Model file for the job. Use its own axes, mm. A direction names the side the tool comes from. Coordinates: 2 decimals unless noted, no trailing zeros. Order: outer loops, then holes, each group sorted by start corner. A loop starts at its lowest first (then second) coordinate and runs counter-clockwise, first axis right, second up.
from build123d import *

# Parameters (mm, degrees)
SKETCH1_R           = 2
SKETCH1_R_2         = 12.51
BOSS_EXTRUDE1_DEPTH = 2
FILLET1_R           = 3
FILLET2_R           = 4.25
FILLET3_R           = 11
CUT_EXTRUDE1_REACH  = 104.947
SKETCH2_R           = 2.25


with BuildPart() as part:
    # Sketch1 → Boss-Extrude1 (new body)
    with BuildSketch(Plane.XY):
        with BuildLine():
            Line((44.023434797, -5), (54, -5))
            Line((54, -5), (54, -19.5))
            Line((54, -19.5), (87, -19.5))
            Line((87, -19.5), (87, -11))
            Line((87, -11), (62.5, -11))
            Line((62.5, -11), (62.5, 30))
            Line((62.5, 30), (87, 30))
            Line((87, 30), (87, 38.5))
            Line((87, 38.5), (55.756354563, 38.5))
            ThreePointArc((55.756354563, 38.5), (41, 45), (26.243645437, 38.5))
            Line((26.243645437, 38.5), (-26.243645437, 38.5))
            ThreePointArc((-26.243645437, 38.5), (-41, 45), (-55.756354563, 38.5))
            Line((-55.756354563, 38.5), (-87, 38.5))
            Line((-87, 38.5), (-87, 30))
            Line((-87, 30), (-62.5, 30))
            Line((-62.5, 30), (-62.5, -11))
            Line((-62.5, -11), (-87, -11))
            Line((-87, -11), (-87, -19.5))
            Line((-87, -19.5), (-54, -19.5))
            Line((-54, -19.5), (-54, -5))
            Line((-54, -5), (-44.723496399, -5))
            Line((-44.723496399, -5), (-10.556829732, -55))
            Line((-10.556829732, -55), (10.704632705, -55))
            Line((10.704632705, -55), (16.51289283, -46.283810101))
            ThreePointArc((16.51289283, -46.283810101), (16.643237983, -46.09065505), (16.771323869, -45.895994479))
            Line((16.771323869, -45.895994479), (44.023434797, -5))
        make_face()
        with Locations((-80, -15.25)):
            Circle(SKETCH1_R, mode=Mode.SUBTRACT)
        with Locations((-70, -15.25)):
            Circle(SKETCH1_R, mode=Mode.SUBTRACT)
        with Locations((0, -35)):
            Circle(SKETCH1_R_2, mode=Mode.SUBTRACT)
        with Locations((70, -15.25)):
            Circle(SKETCH1_R, mode=Mode.SUBTRACT)
        with Locations((80, -15.25)):
            Circle(SKETCH1_R, mode=Mode.SUBTRACT)
        with Locations((-80, 34.25)):
            Circle(SKETCH1_R, mode=Mode.SUBTRACT)
        with Locations((-70, 34.25)):
            Circle(SKETCH1_R, mode=Mode.SUBTRACT)
        with Locations((-41, 25)):
            Circle(SKETCH1_R_2, mode=Mode.SUBTRACT)
        with Locations((41, 25)):
            Circle(SKETCH1_R_2, mode=Mode.SUBTRACT)
        with Locations((70, 34.25)):
            Circle(SKETCH1_R, mode=Mode.SUBTRACT)
        with Locations((80, 34.25)):
            Circle(SKETCH1_R, mode=Mode.SUBTRACT)
    extrude(amount=BOSS_EXTRUDE1_DEPTH)

    # Fillet1
    fillet1_edges = [part.edges().sort_by_distance(p)[0] for p in [
        (62.5, 30, 1),
        (62.5, -11, 1),
        (54, -5, 1),
        (-54, -5, 1),
        (-62.5, -11, 1),
        (-62.5, 30, 1),
    ]]
    fillet(fillet1_edges, radius=FILLET1_R)

    # Fillet2
    fillet2_edges = [part.edges().sort_by_distance(p)[0] for p in [
        (87, 30, 1),
        (87, 38.5, 1),
        (87, -11, 1),
        (87, -19.5, 1),
        (-87, -19.5, 1),
        (-87, -11, 1),
        (-87, 30, 1),
        (-87, 38.5, 1),
        (26.243645437, 38.5, 1),
        (55.756354563, 38.5, 1),
        (-55.756354563, 38.5, 1),
        (-26.243645437, 38.5, 1),
        (44.023434797, -5, 1),
        (-44.723496399, -5, 1),
    ]]
    fillet(fillet2_edges, radius=FILLET2_R - 0.0001)  # a hair under: the kernel refuses the full size

    # Fillet3
    fillet3_edges = [part.edges().sort_by_distance(p)[0] for p in [
        (54, -19.5, 1),
        (-54, -19.5, 1),
    ]]
    fillet(fillet3_edges, radius=FILLET3_R)

    # Sketch2 → Cut-Extrude1 (cut, up to next)
    with BuildSketch(Plane.XY.offset(2), mode=Mode.PRIVATE) as cut_extrude1_sk1:
        with Locations((-41, 41.25)):
            Circle(SKETCH2_R)
    cut_extrude1_tool1 = extrude(cut_extrude1_sk1.sketch, amount=-CUT_EXTRUDE1_REACH, mode=Mode.PRIVATE) & part.part
    # Sketch2 → Cut-Extrude1 (cut, up to next)
    with BuildSketch(Plane.XY.offset(2), mode=Mode.PRIVATE) as cut_extrude1_sk2:
        with Locations((-41, 8.5)):
            Circle(SKETCH2_R)
    cut_extrude1_tool2 = extrude(cut_extrude1_sk2.sketch, amount=-CUT_EXTRUDE1_REACH, mode=Mode.PRIVATE) & part.part
    # Sketch2 → Cut-Extrude1 (cut, up to next)
    with BuildSketch(Plane.XY.offset(2), mode=Mode.PRIVATE) as cut_extrude1_sk3:
        with Locations((41, 8.5)):
            Circle(SKETCH2_R)
    cut_extrude1_tool3 = extrude(cut_extrude1_sk3.sketch, amount=-CUT_EXTRUDE1_REACH, mode=Mode.PRIVATE) & part.part
    # Sketch2 → Cut-Extrude1 (cut, up to next)
    with BuildSketch(Plane.XY.offset(2), mode=Mode.PRIVATE) as cut_extrude1_sk4:
        with Locations((41, 41.5)):
            Circle(SKETCH2_R)
    cut_extrude1_tool4 = extrude(cut_extrude1_sk4.sketch, amount=-CUT_EXTRUDE1_REACH, mode=Mode.PRIVATE) & part.part
    # Sketch2 → Cut-Extrude1 (cut, up to next)
    with BuildSketch(Plane.XY.offset(2), mode=Mode.PRIVATE) as cut_extrude1_sk5:
        with Locations((-16.5, -35)):
            Circle(SKETCH2_R)
    cut_extrude1_tool5 = extrude(cut_extrude1_sk5.sketch, amount=-CUT_EXTRUDE1_REACH, mode=Mode.PRIVATE) & part.part
    # Sketch2 → Cut-Extrude1 (cut, up to next)
    with BuildSketch(Plane.XY.offset(2), mode=Mode.PRIVATE) as cut_extrude1_sk6:
        with Locations((16.5, -35)):
            Circle(SKETCH2_R)
    cut_extrude1_tool6 = extrude(cut_extrude1_sk6.sketch, amount=-CUT_EXTRUDE1_REACH, mode=Mode.PRIVATE) & part.part
    add(cut_extrude1_tool1.solids().sort_by_distance((-41, 41.25, 2))[0], mode=Mode.SUBTRACT)
    add(cut_extrude1_tool2.solids().sort_by_distance((-41, 8.5, 2))[0], mode=Mode.SUBTRACT)
    add(cut_extrude1_tool3.solids().sort_by_distance((41, 8.5, 2))[0], mode=Mode.SUBTRACT)
    add(cut_extrude1_tool4.solids().sort_by_distance((41, 41.5, 2))[0], mode=Mode.SUBTRACT)
    add(cut_extrude1_tool5.solids().sort_by_distance((-16.5, -35, 2))[0], mode=Mode.SUBTRACT)
    add(cut_extrude1_tool6.solids().sort_by_distance((16.5, -35, 2))[0], mode=Mode.SUBTRACT)


solid = part.part
Q1. Cut at A-A, the plane y = 8.5. List the corners of the cut face in (x, z), plus the area to 3 significant figures.
Established:
outline: (-62.5, 0) - (-43.25, 0) - (-43.25, 2) - (-62.5, 2) - close; (-38.75, 0) - (38.75, 0) - (38.75, 2) - (-38.75, 2) - close; (43.25, 0) - (62.5, 0) - (62.5, 2) - (43.25, 2) - close
area: 232 mm2
Q2. Probe line 1 (Y direction, x = -80, z = 0.5); line 2 (Y direction, x = -76, z = 1); line 3 (X direction, y = 22.5, z = 0.3). List the from-to ranges inside material, lowest first.
Established:
line 1: y = -19.5 to -17.25, -13.25 to -11, 30 to 32.25, 36.25 to 38.5
line 2: y = -19.5 to -11, 30 to 38.5
line 3: x = -62.5 to -53.26, -28.74 to 28.74, 53.26 to 62.5
Q3. Mould opens along X. For faces 3 (the face through (57.137, -16.192, 1.014)), 4 (the face through (-85.72, -18.29, 1.01)), 5 (the face through (85.72, 31.21, 1.01)) say: pulls with the +X half, pulls with the -X half, needs draft (parallel to the pull), parting line crosses it, or undercut.
Established:
face 3: undercut
face 4: pulls with the -X half
face 5: pulls with the +X half
Q4. Cut at B-B, the plane x = 48. List the corners of the cut face in (y, z) (3 decimals), plus the area to 3 significant figures.
Established:
outline: (-5, 0) - (14.632, 0) - (14.632, 2) - (-5, 2) - close; (35.368, 0) - (43.735, 0) - (43.735, 2) - (35.368, 2) - close
area: 56.0 mm2
Q5. Drop flat-ended pins along their axis: P1, Ø3, axis at x = 80, y = 34.25, coming from the +Z side; P2, Ø1, axis at x = -51.5, z = 1, coming from the -Y side; P3, Ø1, axis at y = 8, z = 1.5, coming from the +X side; P4, Ø0.6, axis at x = 78, z = 1, coming from the -Y side. Give the stop position or say it passes through.
Established:
P1: passes through
P2: stops at y = -5.17
P3: stops at x = 62.5
P4: stops at y = -19.5
Q6. Which spindle directions (+Z, -Z, +X, -X, +Y, -Y) get a long thin tool onto all of the face, cutting with end or side? Do faces 1 (the face through (-57.137, -16.192, 1.014)), 2 (the face through (52.556, 20.209, 0.986)). Say none if no direction does.
Established:
face 1: +Z, -Z, -Y
face 2: +Z, -Z
Q7. Cut at D-D, the plane z = 1.35. Count the separate pieces of the cut face and the enclosed holes in it, plus the area to 3 significant figures.
Established:
separate pieces: 1
enclosed holes: 17
area: 7,790 mm2
Q8. Cut at C-C, the plane x = -80. List the corners of the cut face in (y, z).
Established:
outline: (-19.5, 0) - (-17.25, 0) - (-17.25, 2) - (-19.5, 2) - close; (-13.25, 0) - (-11, 0) - (-11, 2) - (-13.25, 2) - close; (30, 0) - (32.25, 0) - (32.25, 2) - (30, 2) - close; (36.25, 0) - (38.5, 0) - (38.5, 2) - (36.25, 2) - close
